Build history of the part. All positions in model axes, mm. Coordinates: 2 decimals unless noted, no trailing zeros. Order: outer loops, then holes, each group sorted by start corner. A loop starts at its lowest first (then second) coordinate and runs counter-clockwise, first axis right, second up. Notation, with made-up numbers: (-19, 20) - (6, 20) arc R17 cw to (6, 41) - close; hole circle Ø6 at (-5.5, 19). An arc over 180 degrees is marked (long way). Return JSON: item names as keys, results as strings.
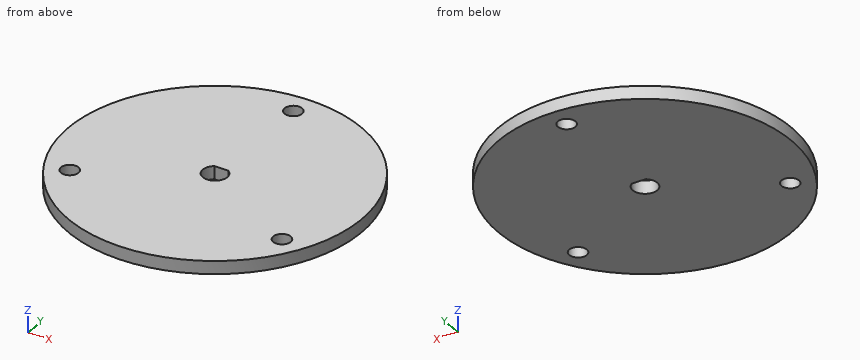
from build123d import *

# Parameters (mm, degrees)
F0_R     = 35.8775
F0_R_2   = 2.15265
F1_DEPTH = 3.175


with BuildPart() as f1:
    # F0 (on Top) → F1 (new body)
    with BuildSketch(Plane.XY):
        Circle(F0_R)
        with Locations((-26.258973, -15.160625)):
            Circle(F0_R_2, mode=Mode.SUBTRACT)
        with BuildLine():
            ThreePointArc((1.715656, 2.460994), (0, -2.999994), (-1.715656, 2.460994))
            Line((-1.715656, 2.460994), (1.715656, 2.460994))
        make_face(mode=Mode.SUBTRACT)
        with Locations((26.258973, -15.160625)):
            Circle(F0_R_2, mode=Mode.SUBTRACT)
        with Locations((0, 30.32125)):
            Circle(F0_R_2, mode=Mode.SUBTRACT)
    extrude(amount=F1_DEPTH)


solid = f1.part
1. Cut at C-C on x = -25. Give the cut face in (y, z) (3 decimals).
Check values:
{"outline": "(-25.733, 0) - (-16.907, 0) - (-16.907, 3.175) - (-25.733, 3.175) - close; (-13.415, 0) - (25.733, 0) - (25.733, 3.175) - (-13.415, 3.175) - close"}
2. Probe L1, parallel to Y at x = 0, z = 2.15; L2, parallel to X at y = -13.5, z = 1.9; L3, parallel to Y at x = -27.5, z = 1.85. List the from-to ranges inside material, lowest first.
Check values:
{"L1": "-35.88 to -3, 2.46 to 28.17, 32.47 to 35.88", "L2": "-33.24 to -27.63, -24.89 to 24.89, 27.63 to 33.24", "L3": "-23.04 to -16.92, -13.4 to 23.04"}
3. Cut at A-A on y = 0. Give the cut face in (x, z) (1 decimal), plus the area to 3 significant figures.
Check values:
{"outline": "(-35.9, 0) - (-3, 0) - (-3, 3.2) - (-35.9, 3.2) - close; (3, 0) - (35.9, 0) - (35.9, 3.2) - (3, 3.2) - close", "area": "209 mm²"}
4. Drop flat-ended pins along their axis: pin 1 (1.5 mm diameter, centred on y = -27, z = 0.5, fed in from +X); pin 2 (1.6 mm diameter, centred on x = 0, z = 1.5, fed in from -Y); pin 3 (1.5 mm diameter, centred on y = 2, z = 2.5, fed in from -X). Give the stop position or say it passes through.
Check values:
{"pin 1": "x = 24.46", "pin 2": "y = -35.88", "pin 3": "x = -35.86"}
5. Cut at D-D on y = -14. Give the cut face in (x, z) (3 decimals), plus the area to 3 significant figures.
Check values:
{"outline": "(-33.033, 0) - (-28.072, 0) - (-28.072, 3.175) - (-33.033, 3.175) - close; (-24.446, 0) - (24.446, 0) - (24.446, 3.175) - (-24.446, 3.175) - close; (28.072, 0) - (33.033, 0) - (33.033, 3.175) - (28.072, 3.175) - close", "area": "187 mm²"}
6. Cut at B-B on x = 0. Give the cut face in (y, z) (1 decimal), plus the area to 3 significant figures.
Check values:
{"outline": "(-35.9, 0) - (-3, 0) - (-3, 3.2) - (-35.9, 3.2) - close; (2.5, 0) - (28.2, 0) - (28.2, 3.2) - (2.5, 3.2) - close; (32.5, 0) - (35.9, 0) - (35.9, 3.2) - (32.5, 3.2) - close", "area": "197 mm²"}
